```python
from build123d import *

# Parameters (mm, degrees)
F1_DEPTH = 30
F2_R     = 4
F2_W     = 8
F2_H     = 50
F3_DEPTH = 30.001
F4_R     = 4
F5_DEPTH = 30.001
F7_DEPTH = 30.001


with BuildPart() as f1:
    # F0 (on Front) → F1 (new body)
    with BuildSketch(Plane.XZ):
        Polygon((15, 30), (-15, 30), (-15, -30), (-6, -30), (-6, 0), (6, 0), (6, -30), (15, -30), align=None)
    extrude(amount=F1_DEPTH)

    # F2 (on face) → F3 (cut, through all)
    with BuildSketch(Plane(origin=(-15, 0, 0), x_dir=(0, -1, 0), z_dir=(-1, 0, 0))):
        with Locations((14.645997, -14.849633)):
            Circle(F2_R)
        with Locations((15, 30)):
            Rectangle(F2_W, F2_H)
    extrude(amount=-F3_DEPTH, mode=Mode.SUBTRACT)

    # F4 (on face) → F5 (cut, through all)
    with BuildSketch(Plane(origin=(0, 0, 0), x_dir=(-1, 0, 0), z_dir=(0, 1, 0))):
        with Locations((0, 14.751268)):
            Circle(F4_R)
    extrude(amount=-F5_DEPTH, mode=Mode.SUBTRACT)

    # F6 (on face) → F7 (cut, through all)
    with BuildSketch(Plane(origin=(0, 0, 0), x_dir=(-1, 0, 0), z_dir=(0, 1, 0))):
        with BuildLine():
            ThreePointArc((0, 30), (9.76466, 26.463451), (15, 17.494227))
            Line((15, 17.494227), (15, 30))
            Line((15, 30), (0, 30))
        make_face()
        with BuildLine():
            ThreePointArc((-15, 17.494227), (-9.76466, 26.463451), (0, 30))
            Line((0, 30), (-15, 30))
            Line((-15, 30), (-15, 17.494227))
        make_face()
    extrude(amount=-F7_DEPTH, mode=Mode.SUBTRACT)


solid = f1.part
```
The model under review builds one solid part; all positions refer to its coordinate system, in mm. A direction names the side the tool comes from. Give positions to 0.01 mm unless a question says otherwise; leave off trailing zeros. Write each loop counter-clockwise with the first axis right and the second up, starting at its lowest first coordinate (ties: lowest second). Pieces come first, ordered by that corner, then holes. Notation, with made-up numbers: M 38.25,-27.5 L 91.25,-27.5 A14 ccw 91.25,-11.5 Z; hole C 89,42 d6. An arc over 180 degrees is marked long. Write each question's results on one line, items separated by ' | '. Start each with the question number.
1. We need section D-D (y = -4.75). Write out the cut boundary in (x, z), and give its area (3 significant figures).
2. We need section C-C (x = 2.5). Write out the cut boundary in (y, z).
3. For probe 1 along Z at (x, y) = (0, -6.25); probe 2 along Y at (x, z) = (4, 16); probe 3 along X at (y, z) = (-7.5, -27), list the stretches that pass through material, from the lowest coordinate up. Write a range as [from, to].
4. We need section A-A (z = 8). Write out the cut boundary in (x, y), and give its area (3 significant figures).
5. For faces 4 (the flat face through (6, -18, -11)), 5 (the flat face through (10, -15, -30)), 6 (the flat face through (0, -15, 5)), list the 3-axis set-ups (+Z, -Z, +X, -X, +Y, -Y) from which the entire face can be reached by the end or side of a thin tool; tool diameter is ignored.
6. We need section B-B (x = -7.25). Write out the cut boundary in (y, z), and give its area (3 significant figures).
7. Insertion check: pin 1 Ø2 at (y, z) = (-8.5, 24) entering from +X; pin 2 Ø7 at (x, z) = (0, 14.75) entering from +Y; pin 3 Ø1.5 at (y, z) = (-19, 21) entering from -X. Each pin has a flat end and moves straight along its axis. Give the tip position at first contact, or say it passes through.
8. Mouldability with a two-part tool opening along X and no side actions: class faces 1 (the flat face through (-4, -19, 17)), 2 (the flat face through (15, -15, -7)), 3 (the flat face through (-6, -18, -19)) as released by +X, released by -X, zero draft, split by the parting line, or undercut.
Results found:
1) outline: M -15,-30 L -6,-30 L -6,0 L 6,0 L 6,-30 L 15,-30 L 15,17.49 A15.25 ccw 0,30 A15.25 ccw -15,17.49 Z; hole C 0,14.75 d8 | area: 1,300 mm^2
2) outline: M -30,0 L 0,0 L 0,11.63 L -11,11.63 L -11,5 L -19,5 L -19,11.63 L -30,11.63 Z; M -30,17.87 L -19,17.87 L -19,29.79 L -30,29.79 Z; M -11,17.87 L 0,17.87 L 0,29.79 L -11,29.79 Z
3) probe 1: z = [0, 10.75], [18.75, 30] | probe 2: y = [-30, -19], [-11, 0] | probe 3: x = [-15, -6], [6, 15]
4) outline: M -15,-30 L 15,-30 L 15,-19 L -15,-19 Z; M -15,-11 L 15,-11 L 15,0 L -15,0 Z | area: 660 mm^2
5) face 4: -Z, +Y, -Y | face 5: -Z, +X, -X, +Y, -Y | face 6: +Z, +X, -X
6) outline: M -30,-30 L 0,-30 L 0,28.17 L -11,28.17 L -11,5 L -19,5 L -19,28.17 L -30,28.17 Z; hole C -14.65,-14.85 d8 | area: 1,510 mm^2
7) pin 1: stops at x = 12.83 | pin 2: passes through | pin 3: stops at x = -14.22
8) face 1: zero draft | face 2: released by +X | face 3: undercut
